Geometry: final body of the model. Coordinates: model frame, mm. A direction names the side the tool comes from. Coordinates: 2 decimals unless noted, no trailing zeros. Order: outer loops, then holes, each group sorted by start corner. A loop starts at its lowest first (then second) coordinate and runs counter-clockwise, first axis right, second up. Notation, with made-up numbers: M -29.75,37 L 16.25,37 A25 ccw 16.25,59 Z; hole C -8.5,-13 d4. An arc over 180 degrees is marked long. Write item = value, one per line.
from build123d import *

# Parameters (mm, degrees)
SKETCH1_W           = 150
SKETCH1_H           = 30
BOSS_EXTRUDE1_DEPTH = 10
CUT_EXTRUDE1_DEPTH  = 10
SKETCH2_3_W         = 15.5
SKETCH2_3_H         = 23
BOSS_EXTRUDE2_DEPTH = 20
FILLET1_R           = 5


with BuildPart() as part:
    # Sketch1 → Boss-Extrude1 (new body)
    with BuildSketch(Plane(origin=(0, 0, 0), x_dir=(1, 0, 0), z_dir=(0, 1, 0))):
        Rectangle(SKETCH1_W, SKETCH1_H)
    extrude(amount=BOSS_EXTRUDE1_DEPTH)

    # Sketch2 → Cut-Extrude1 (cut)
    with BuildSketch(Plane(origin=(0, 10, 0), x_dir=(1, 0, 0), z_dir=(0, 1, 0))):
        Polygon((-60.3, -12), (-60.3, -15), (-50.8, -15), (-50.8, -12), (-50.8, 5), (-60.3, 5), align=None)
        Polygon((50.8, -15), (60.3, -15), (60.3, -12), (60.3, 5), (50.8, 5), (50.8, -12), align=None)
    extrude(amount=-CUT_EXTRUDE1_DEPTH, mode=Mode.SUBTRACT)

    # Sketch2_3 → Boss-Extrude2 (add)
    with BuildSketch(Plane(origin=(0, 10, 0), x_dir=(1, 0, 0), z_dir=(0, 1, 0))):
        Polygon((-63.3, 8), (-63.3, -15), (-60.3, -15), (-60.3, -12), (-60.3, 5), (-50.8, 5), (-50.8, -12), (-50.8, -15), (-47.8, -15), (-47.8, 8), align=None)
        with Locations((-25.05, -3.5)):
            Rectangle(SKETCH2_3_W, SKETCH2_3_H)
        with Locations((25.05, -3.5)):
            Rectangle(SKETCH2_3_W, SKETCH2_3_H)
        Polygon((47.8, 8), (47.8, -15), (50.8, -15), (50.8, -12), (50.8, 5), (60.3, 5), (60.3, -12), (60.3, -15), (63.3, -15), (63.3, 8), align=None)
    extrude(amount=BOSS_EXTRUDE2_DEPTH)

    # Fillet1
    fillet1_edges = [part.edges().sort_by_distance(p)[0] for p in [
        (0, 0, -15),
    ]]
    fillet(fillet1_edges, radius=FILLET1_R)


solid = part.part
1) Section B-B, the plane y = 19.5. Return loops of the section in (x, z), and give its area (3 significant figures).
Numbers:
outline = M -63.3,-8 L -47.8,-8 L -47.8,15 L -50.8,15 L -50.8,-5 L -60.3,-5 L -60.3,15 L -63.3,15 Z; M -32.8,-8 L -17.3,-8 L -17.3,15 L -32.8,15 Z; M 17.3,-8 L 32.8,-8 L 32.8,15 L 17.3,15 Z; M 47.8,-8 L 63.3,-8 L 63.3,15 L 60.3,15 L 60.3,-5 L 50.8,-5 L 50.8,15 L 47.8,15 Z
area = 1,050 mm²
2) Line query: L1, parallel to X at y = 7.25, z = 2.75; L2, parallel to X at y = 24, z = 5; L3, parallel to Y at x = -38, z = -6. Output: solid intervals per line, ascending.
Numbers:
L1 = -75 to -60.3, -50.8 to 50.8, 60.3 to 75
L2 = -63.3 to -60.3, -50.8 to -47.8, -32.8 to -17.3, 17.3 to 32.8, 47.8 to 50.8, 60.3 to 63.3
L3 = 0 to 10
3) Section D-D, the plane y = 8. Return loops of the section in (x, z), and give its area (3 significant figures).
Numbers:
outline = M -75,-15 L 75,-15 L 75,15 L 60.3,15 L 60.3,-5 L 50.8,-5 L 50.8,15 L -50.8,15 L -50.8,-5 L -60.3,-5 L -60.3,15 L -75,15 Z
area = 4,120 mm²
4) Section C-C, the plane x = 29. Return loops of the section in (y, z), and give its area (3 significant figures).
Numbers:
outline = M 0,-10 A5 ccw 5,-15 L 10,-15 L 10,-8 L 30,-8 L 30,15 L 0,15 Z
area = 755 mm²
5) Mould query, pull axis X, two halves, no side actions, for faces 1 (the face through (1, 2, -14)), 2 (the face through (-75, 5, 0)), 3 (the face through (32.8, 20, 4)), 4 (the face through (-47.8, 20, 4)). Classes: pulls with the +X half, pulls with the -X half, needs draft (parallel to the pull), parting line crosses it, or undercut.
Numbers:
face_1 = needs draft
face_2 = pulls with the -X half
face_3 = undercut
face_4 = undercut
6) Pin query (flat end, axial travel): pin 1 (8 mm diameter, centred on x = 31, z = 0, fed in from -Y); pin 2 (5 mm diameter, centred on x = -24.5, y = 15, fed in from -Z); pin 3 (10 mm diameter, centred on y = 23, z = 8, fed in from -X); pin 4 (4 mm diameter, centred on x = 3.5, z = 1, fed in from +Y). Return the tip coordinate at first contact, or that it passes through.
Numbers:
pin_1 = 0
pin_2 = -8
pin_3 = -63.3
pin_4 = 10
7) Set-up query: faces 5 (the face through (47.8, 20, 3)), 6 (the face through (-56, 15, -5)), 7 (the face through (-63.3, 20, 3)), 8 (the face through (63.3, 20, 4)), 9 (the face through (25, 20, -8)). Return all of +Z, -Z, +X, -X, +Y, -Y with unobstructed straight access to the full face (end or side cutting, diameter ignored); none if empty.
Numbers:
face_5 = +Z, -Z, +Y
face_6 = +Z, +Y, -Y
face_7 = +Z, -Z, -X, +Y
face_8 = +Z, -Z, +X, +Y
face_9 = -Z, +X, -X, +Y
8) Section A-A, the plane z = 2.75. Return loops of the section in (x, y).
Numbers:
outline = M -75,0 L -60.3,0 L -60.3,30 L -63.3,30 L -63.3,10 L -75,10 Z; M -50.8,0 L 50.8,0 L 50.8,30 L 47.8,30 L 47.8,10 L 32.8,10 L 32.8,30 L 17.3,30 L 17.3,10 L -17.3,10 L -17.3,30 L -32.8,30 L -32.8,10 L -47.8,10 L -47.8,30 L -50.8,30 Z; M 60.3,0 L 75,0 L 75,10 L 63.3,10 L 63.3,30 L 60.3,30 Z
